Can you work these out from the model? Positions are in its coordinate system, mm. A direction names the side the tool comes from. Give positions to 0.01 mm unless a question says otherwise; leave off trailing zeros. Order: outer loops, then holes, each group sorted by start corner. A loop starts at its lowest first (then second) coordinate and runs counter-clockwise, first axis right, second up. Notation, with made-up numbers: (-1, -13.75) - (30, -13.75) arc R24 cw to (30, 5.25) - close; hole circle Ø9 at (55.5, 53.25). An arc over 180 degrees is marked (long way). Use one line per item in the form item = value. Start each with the question number.
1) We'd pull the mould along X, two halves only. Please class faces 6 (the flat face through (6.5, 46, 33)), 7 (the flat face through (0, -56, 6)), 8 (the flat face through (-24, 9, 21)): released by +X, released by -X, zero draft, split by the parting line, or undercut.
2) Suppose I cut it at D-D, the plane y = -43.5. Write out the boundary of the cut face in (x, z).
3) Please list where these lines run through material, in increasing order: probe 1 along Y at (x, z) = (-11, 8.75); probe 2 along Y at (x, z) = (-8, 4); probe 3 along X at (y, z) = (40.5, 34).
4) Which directions (+Z, -Z, +X, -X, +Y, -Y) give clear straight access to the entire face, cutting with the end or side of a thin tool? Please do faces 1 (the flat face through (0, 51, 16)), 2 (the flat face through (0, -42, 11)), 3 (the cylindrical face through (0.1, 45.6, 18.5)), 4 (the flat face through (0, -38, 0)), 5 (the flat face through (0, 34, 11)).
5) For pin 1 (9 mm diameter, centred on x = -1.5, z = 21.5, fed in from -Y); pin 2 (2 mm diameter, centred on y = 23, z = 23, fed in from -X); pin 3 (13 mm diameter, centred on x = 11, y = -41.96, fed in from +Z); pin 4 (2 mm diameter, centred on x = 0, z = 27.5, fed in from +Y), each with a flat end and sliding along its axis, tell me the tip position at first contact or that it passes through.
6) Suppose I cut it at C-C, the plane x = 0. Write out the boundary of the cut face in (y, z).
7) Suppose I cut it at B-B, the plane z = 37. Write out the boundary of the cut face in (x, y).
8) Suppose I cut it at A-A, the plane y = 0. Write out the boundary of the cut face in (x, z), and give its area (3 significant figures).
```python
from build123d import *

# Parameters (mm, degrees)
F0_W     = 11
F0_H     = 30
F1_DEPTH = 24
F3_DEPTH = 17.9
F4_R     = 5
F4_R_2   = 2.5
F5_DEPTH = 51.2


with BuildPart() as f1:
    # F0 (on Right) → F1 (new body, symmetric)
    with BuildSketch(Plane.YZ):
        with BuildLine():
            Line((-56, 0), (-30, 0))
            ThreePointArc((-30, 0), (-29.4730143031, 5.5983415304), (-27.9105714739, 11))
            Line((-27.9105714739, 11), (-56, 11))
            Line((-56, 11), (-56, 0))
        make_face()
        with BuildLine():
            ThreePointArc((-27.9105714739, 11), (-29.4730143031, 5.5983415304), (-30, 0))
            Line((-30, 0), (-19, 0))
            ThreePointArc((-19, 0), (-18.1017503893, 5.7729223833), (-15.4919333848, 11))
            Line((-15.4919333848, 11), (-27.9105714739, 11))
        make_face()
        with BuildLine():
            Line((15.4919333848, 11), (27.9105714739, 11))
            ThreePointArc((27.9105714739, 11), (0, 30), (-27.9105714739, 11))
            Line((-27.9105714739, 11), (-15.4919333848, 11))
            ThreePointArc((-15.4919333848, 11), (0, 19), (15.4919333848, 11))
        make_face()
        with BuildLine():
            Line((19, 0), (30, 0))
            ThreePointArc((30, 0), (29.4730143031, 5.5983415304), (27.9105714739, 11))
            Line((27.9105714739, 11), (15.4919333848, 11))
            ThreePointArc((15.4919333848, 11), (18.1017503893, 5.7729223833), (19, 0))
        make_face()
        with BuildLine():
            ThreePointArc((27.9105714739, 11), (29.4730143031, 5.5983415304), (30, 0))
            Line((30, 0), (51, 0))
            Line((51, 0), (51, 11))
            Line((51, 11), (40, 11))
            Line((40, 11), (27.9105714739, 11))
        make_face()
        with Locations((45.5, 26)):
            Rectangle(F0_W, F0_H)
    extrude(amount=F1_DEPTH, both=True)

    # F2 (on face) → F3 (cut, symmetric)
    with BuildSketch(Plane(origin=(0, 51, 0), x_dir=(-1, 0, 0), z_dir=(0, 1, 0))):
        with BuildLine():
            ThreePointArc((-6.5, 25), (0, 18.5), (6.5, 25))
            ThreePointArc((6.5, 25), (0, 31.5), (-6.5, 25))
        make_face()
        with BuildLine():
            ThreePointArc((-6.5, 25), (0, 31.5), (6.5, 25))
            Line((6.5, 25), (6.5, 41))
            Line((6.5, 41), (-6.5, 41))
            Line((-6.5, 41), (-6.5, 25))
        make_face()
    extrude(amount=F3_DEPTH, both=True, mode=Mode.SUBTRACT)

    # F4 (on Top) → F5 (cut, symmetric)
    with BuildSketch(Plane.XY):
        with Locations((-11, -41.955285737)):
            Circle(F4_R)
        with Locations((11, -41.955285737)):
            Circle(F4_R)
        Circle(F4_R_2)
    extrude(amount=F5_DEPTH, both=True, mode=Mode.SUBTRACT)


solid = f1.part
```
Result sheet:
q1.face_6 = undercut
q1.face_7 = zero draft
q1.face_8 = released by -X
q2.outline = (-24, 0) - (-15.76, 0) - (-15.76, 11) - (-24, 11) - close; (-6.24, 0) - (6.24, 0) - (6.24, 11) - (-6.24, 11) - close; (15.76, 0) - (24, 0) - (24, 11) - (15.76, 11) - close
q3.probe_1 = -56 to -46.96, -36.96 to -16.87, 16.87 to 51
q3.probe_2 = -56 to -45.96, -37.96 to -18.57, 18.57 to 51
q3.probe_3 = -24 to -6.5, 6.5 to 24
q4.face_1 = +Z, -Z, +X, -X, +Y
q4.face_2 = +Z, +X, -X, -Y
q4.face_3 = +Z, +Y
q4.face_4 = -Z, +X, -X, +Y, -Y
q4.face_5 = +Z, +X, -X
q5.pin_1 = -24.72
q5.pin_2 = through
q5.pin_3 = 11
q5.pin_4 = 14.06
q6.outline = (-56, 0) - (-19, 0) arc R19 cw to (-2.5, 18.83) - (-2.5, 29.9) arc R30 ccw to (-27.91, 11) - (-56, 11) - close; (2.5, 18.83) arc R19 cw to (19, 0) - (51, 0) - (51, 18.5) - (40, 18.5) - (40, 11) - (27.91, 11) arc R30 ccw to (2.5, 29.9) - close
q7.outline = (-24, 40) - (-6.5, 40) - (-6.5, 51) - (-24, 51) - close; (6.5, 40) - (24, 40) - (24, 51) - (6.5, 51) - close
q8.outline = (-24, 19) - (-2.5, 19) - (-2.5, 30) - (-24, 30) - close; (2.5, 19) - (24, 19) - (24, 30) - (2.5, 30) - close
q8.area = 473 mm²
